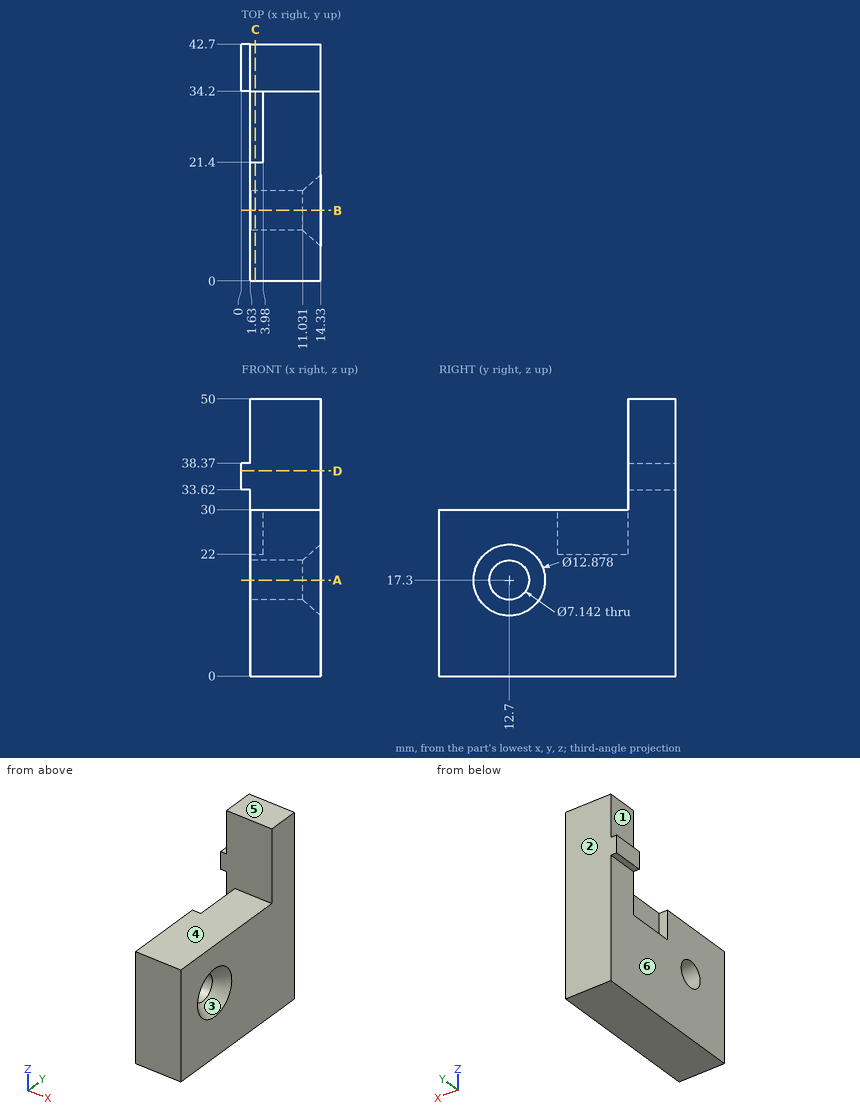
Geometry check sheet. Reference: drawing and pictorial views, mm from the part's lowest x, y, z. A direction names the side the tool comes from. Coordinates: 2 decimals unless noted, no trailing zeros. Write each loop counter-clockwise with the first axis right and the second up, starting at its lowest first coordinate (ties: lowest second). Pieces come first, ordered by that corner, then holes. Notation, with made-up numbers: M 16,76 L 52,76 A16 cw 52,95 Z; hole C 14,74.5 d10. An arc over 180 degrees is marked long. Write item = value, one per line. Start each with the question number.
1. Sectioned sample at A-A (z = 17.3). Record the cut outline in (x, y).
2. Tool access check on the marked faces 4, 5 and 6. Record the directions out of +Z, -Z, +X, -X, +Y, -Y that give a thin tool (end or side, any length) a straight path to the whole face; none if there is none.
3. Mould release check, pull along Y, two halves, no side actions. Record for the marked faces 1, 2 and 3: pulls with the +Y half, pulls with the -Y half, needs draft (parallel to the pull), parting line crosses it, or undercut.
4. Sectioned sample at C-C (x = 2.5). Record the cut outline in (y, z).
5. Go/stop test with flat-tipped pins: pin 1 (6 mm diameter, centred on y = 4.5, z = 27, fed in from -X); pin 2 (0.8 mm diameter, centred on x = 0.5, y = 37.5, fed in from -Z); pin 3 (8 mm diameter, centred on y = 12.7, z = 17.3, fed in from +X) (1 decimal); pin 4 (8 mm diameter, centred on x = 11.5, y = 24, fed in from -Z). Record where each tip stops, or that it passes through.
6. Sectioned sample at D-D (z = 37). Record the cut outline in (x, y), then the cut area to 3 significant figures.
7. Sectioned sample at B-B (y = 12.7). Record the cut outline in (x, z).
8. Thickness scan on probe 1 along Y at (x, z) = (8.75, 17.3); probe 2 along Z at (x, y) = (7.75, 4); probe 3 along Y at (x, z) = (4.5, 45.5). Record the ranges inside material, lowest first.
The answers:
q1.outline = M 1.63,0 L 14.33,0 L 14.33,6.26 L 11.03,9.13 L 1.63,9.13 Z; M 1.63,16.27 L 11.03,16.27 L 14.33,19.14 L 14.33,42.7 L 1.63,42.7 Z
q2.face_4 = +Z, +X, -X, -Y
q2.face_5 = +Z, +X, -X, +Y, -Y
q2.face_6 = -Z, -X, +Y, -Y
q3.face_1 = needs draft
q3.face_2 = pulls with the +Y half
q3.face_3 = undercut
q4.outline = M 0,0 L 42.7,0 L 42.7,50 L 34.2,50 L 34.2,22 L 21.4,22 L 21.4,30 L 0,30 Z; hole C 12.7,17.3 d7.14
q5.pin_1 = 1.63
q5.pin_2 = 33.62
q5.pin_3 = 11.5
q5.pin_4 = 0
q6.outline = M 0,34.2 L 14.33,34.2 L 14.33,42.7 L 0,42.7 Z
q6.area = 122 mm²
q7.outline = M 1.63,0 L 14.33,0 L 14.33,10.86 L 11.03,13.73 L 1.63,13.73 Z; M 1.63,20.87 L 11.03,20.87 L 14.33,23.74 L 14.33,30 L 1.63,30 Z
q8.probe_1 = 0 to 9.13, 16.27 to 42.7
q8.probe_2 = 0 to 30
q8.probe_3 = 34.2 to 42.7
